```python
from build123d import *

# Parameters (mm, degrees)
F0_W      = 152.4
F0_H      = 38.1
F3_R      = 31.75
F4_DEPTH  = 25.4
F5_DEPTH  = 50.8
F7_DEPTH  = 76.2
F11_DEPTH = 76.2
F12_R     = 28.575
F13_DEPTH = 146.05
F14_R     = 9.525
F15_DEPTH = 50.8
F17_D     = 4.826
F17_DEPTH = 12.7
F17_TIP   = 1.4498766737
F19_D     = 12.7
F19_DEPTH = 12.7
F19_TIP   = 3.8154649308


# Not quite as in the source:
# - a feature names something its author has since deleted; it is built from what else it names


with BuildPart() as f1:
    # F0 (on Front) → F1 (revolve)
    with BuildSketch(Plane.XZ):
        with Locations((76.2, 19.05)):
            Rectangle(F0_W, F0_H)
    revolve(axis=Axis((76.2, 0, 0), (1, 0, 0)))

    # F3 (on offset) → F4 (join)
    with BuildSketch(Plane.XY.offset(38.1)):
        with Locations((107.95, 0)):
            Circle(F3_R)
    extrude(amount=-F4_DEPTH)

    # F5 (add): a face of the model
    f5_faces = [f1.faces().sort_by_distance(p)[0] for p in [
        (107.95, 0, 38.1),
    ]]
    extrude(f5_faces, amount=F5_DEPTH)

    # F6 (on face) → F7 (join)
    with BuildSketch(Plane.XY.offset(88.9)):
        with BuildLine():
            Line((73.025, -22.0412760045), (85.097327244, -22.0412760045))
            ThreePointArc((85.097327244, -22.0412760045), (76.2, 0), (85.097327244, 22.0412760045))
            Line((85.097327244, 22.0412760045), (73.025, 22.0412760045))
            Line((73.025, 22.0412760045), (73.025, -22.0412760045))
        make_face()
    extrude(amount=-F7_DEPTH)

    # F8 (on Front) → F9 (revolve)
    with BuildSketch(Plane.XZ):
        Polygon((33.2235226281, 67.1248349075), (22.225, 60.7748349075), (38.982496247, 31.75), (49.9810188751, 38.1), align=None)
    revolve(axis=Axis((30.6037481235, 0, 46.2624174538), (0.5, 0, -0.8660254038)))

    # F10 (on face) → F11 (cut)
    with BuildSketch(Plane.XY.offset(88.9)):
        with BuildLine():
            Line((79.3750002146, -15.69127579), (87.9764211223, -15.69127579))
            ThreePointArc((87.9764211223, -15.69127579), (133.3499997854, 0), (87.9764211223, 15.69127579))
            Line((87.9764211223, 15.69127579), (79.3750002146, 15.69127579))
            Line((79.3750002146, 15.69127579), (79.3750002146, -15.69127579))
        make_face()
    extrude(amount=-F11_DEPTH, mode=Mode.SUBTRACT)

    # F12 (on face) → F13 (cut)
    with BuildSketch(Plane.YZ.offset(152.4)):
        Circle(F12_R)
    extrude(amount=-F13_DEPTH, mode=Mode.SUBTRACT)

    # F14 (on face) → F15 (cut)
    with BuildSketch(Plane(origin=(-20.7600254704, 0, 35.9574188811), x_dir=(0.8660254038, 0, 0.5), z_dir=(-0.5, 0, 0.8660254038))):
        with Locations((49.6348320529, 0)):
            Circle(F14_R)
    extrude(amount=-F15_DEPTH, mode=Mode.SUBTRACT)

    # F17
    with Locations(Plane.YZ.offset(152.4)):
        with Locations((-23.8125, 23.8125), (23.8125, 23.8125), (23.8125, -23.8125), (-23.8125, -23.8125)):
            Hole(F17_D / 2, depth=F17_DEPTH)
            with Locations((0, 0, -(F17_DEPTH + F17_TIP / 2))):  # 118° drill point
                Cone(0, F17_D / 2, F17_TIP, mode=Mode.SUBTRACT)

    # F19
    with Locations(Plane(origin=(0, 0, 0), x_dir=(0, -1, 0), z_dir=(-1, 0, 0))):
        with Locations((0, 0)):
            Hole(F19_D / 2, depth=F19_DEPTH)
            with Locations((0, 0, -(F19_DEPTH + F19_TIP / 2))):  # 118° drill point
                Cone(0, F19_D / 2, F19_TIP, mode=Mode.SUBTRACT)


solid = f1.part
```
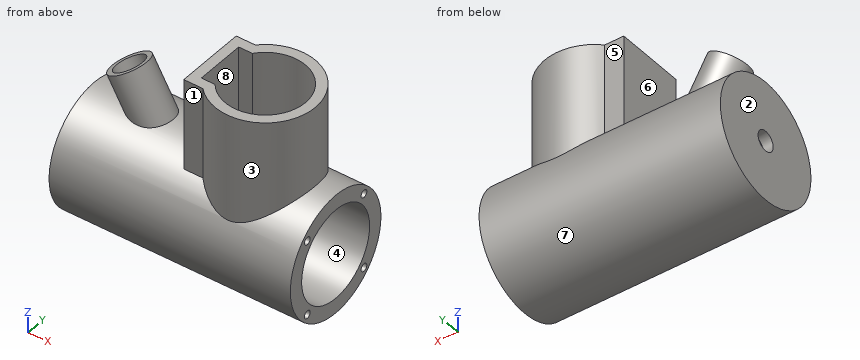
The listing builds one solid part. Answer for the finished solid, in the listing's coordinates (mm). Face numbers are marked on the shaded views. A direction names the side the tool comes from. Round coordinates to 2 decimals unless told otherwise and drop trailing zeros. Loops run counter-clockwise (first coordinate to the right, second up) from the corner with the lowest first, then second, coordinate; pieces in that order, holes last. Notation, with made-up numbers: (-1, 77.5) - (56, 77.5) arc R26 ccw to (56, 99.5) - close; hole circle Ø4 at (-18, -2.5). An arc over 180 degrees is marked (long way). Return JSON: item names as keys, results as strings. Group by question number.
1. The part is cut by section B-B on z = 76.5. Determine the outline of the cut face in (x, y) (3 decimals), then the cut area to 3 significant figures.
2. The mould has two halves that part along Y. Classify the marked faces 6, 7 and 8: pulls with the +Y half, pulls with the -Y half, needs draft (parallel to the pull), parting line crosses it, or undercut.
3. Consider probe 1 along Y at (x, z) = (83, 68); probe 2 along Y at (x, z) = (108.5, 27.5); probe 3 along Z at (x, y) = (3.5, 0). Determine where each line is inside the solid, lowest interval first.
4. The part is cut by section C-C on y = 18. Determine the outline of the cut face in (x, z) (3 decimals).
5. The part is cut by section D-D on x = 107.95. Determine the outline of the cut face in (y, z) (3 decimals), then the cut area to 3 significant figures.
6. Each of these flat-tipped pins is pushed along its axis until it touches: P1, Ø13.5, axis at x = 81.5, z = 53, coming from the +Y side; P2, Ø13, axis at y = -4.5, z = 59.5, coming from the -X side; P3, Ø10, axis at x = 132, y = 26.5, coming from the -Z side. Where does it stop, or does it pass through?
7. Which of the six approach directions +Z, -Z, +X, -X, +Y, -Y give full straight-line access (tool end or side, diameter ignored) to the marked faces 1, 2, 3, 4 and 5?
8. The part is cut by section A-A on z = 0. Determine the outline of the cut face in (x, y) (3 decimals), then the cut area to 3 significant figures.
Resolved:
{
 "1": {"outline": "(73.025, -22.041) - (85.097, -22.041) arc R31.75 ccw (long way) to (85.097, 22.041) - (73.025, 22.041) - close; hole (79.375, -15.691) - (87.976, -15.691) arc R25.4 ccw (long way) to (87.976, 15.691) - (79.375, 15.691) - close", "area": "1,250 mm²"},
 "2": {"face 6": "needs draft", "face 7": "parting line crosses it", "face 8": "undercut"},
 "3": {"probe 1": "y = -22.04 to -15.69, 15.69 to 22.04", "probe 2": "y = -31.75 to -25.39, 25.39 to 31.75", "probe 3": "z = -38.1 to -6.35, 6.35 to 38.1"},
 "4": {"outline": "(0, -33.58) - (152.4, -33.58) - (152.4, -22.193) - (6.35, -22.193) - (6.35, 22.193) - (90.029, 22.193) - (90.029, 88.9) - (73.025, 88.9) - (73.025, 33.58) - (0, 33.58) - close; (125.871, 22.193) - (152.4, 22.193) - (152.4, 33.58) - (134.105, 33.58) - (134.105, 88.9) - (125.871, 88.9) - close"},
 "5": {"outline": "(-31.75, 21.061) arc R38.1 ccw (long way) to (31.75, 21.061) - (31.75, 88.9) - (25.4, 88.9) - (25.4, 13.091) arc R28.575 cw (long way) to (-25.4, 13.091) - (-25.4, 88.9) - (-31.75, 88.9) - close", "area": "2,250 mm²"},
 "6": {"P1": "stops at y = 24.9", "P2": "stops at x = 11.23", "P3": "stops at z = -31.45"},
 "7": {"face 1": "+Z, -X, -Y", "face 2": "+Z, -Z, -X, +Y, -Y", "face 3": "+Z", "face 4": "+X", "face 5": "+Z, -X, +Y"},
 "8": {"outline": "(0, -38.1) - (152.4, -38.1) - (152.4, -28.575) - (6.35, -28.575) - (6.35, -6.35) - (0, -6.35) - close; (0, 6.35) - (6.35, 6.35) - (6.35, 28.575) - (152.4, 28.575) - (152.4, 38.1) - (0, 38.1) - close", "area": "3,190 mm²"}
}
